CAD build for the part. Positions are in the model's coordinates, mm. Face numbers are marked on the shaded views. A direction names the side the tool comes from. Round coordinates to 2 decimals unless told otherwise and drop trailing zeros. Loops run counter-clockwise (first coordinate to the right, second up) from the corner with the lowest first, then second, coordinate; pieces in that order, holes last. Notation, with made-up numbers: M 23,64 L 34,64 A22 ccw 34,89 Z; hole C -24,-20 d10. An arc over 180 degrees is marked long. One line per item, written item: value. Start each with the question number.
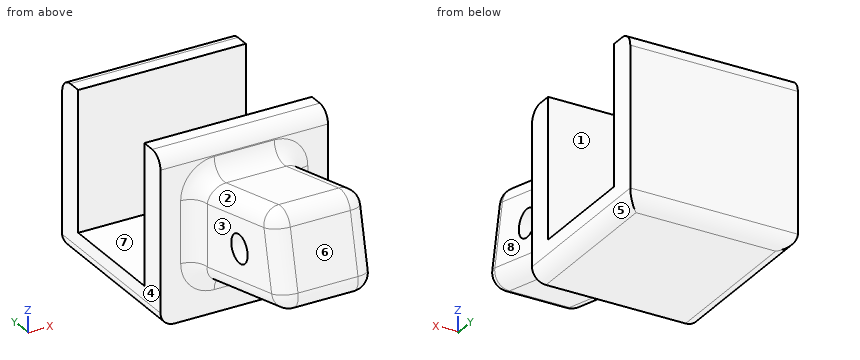
from build123d import *

# Parameters (mm, degrees)
F0_W      = 30
F0_H      = 30
F1_DEPTH  = 5
F2_W      = 30
F2_H      = 4.9
F3_DEPTH  = 25
F6_W      = 16.75
F6_H      = 16.75
F7_DEPTH  = 25
F7_FACE_W = 16.75
F7_FACE_H = 8.375
F9_R      = 3
F10_R     = 2.5
F12_R     = 2.5
F13_DEPTH = 16.75


# Not quite as in the source:
# - two fillets or chamfers of one size are made in one step
# - a feature names something its author has since deleted; it is built from what else it names


with BuildPart() as f1:
    # F0 (on Top) → F1 (new body)
    with BuildSketch(Plane.XY):
        with Locations((15, 15)):
            Rectangle(F0_W, F0_H)
    extrude(amount=F1_DEPTH)

    # F2 (on face) → F3 (join)
    with BuildSketch(Plane.XY.offset(5)):
        with Locations((15, 27.55)):
            Rectangle(F2_W, F2_H)
        with Locations((15, 2.45)):
            Rectangle(F2_W, F2_H)
    extrude(amount=F3_DEPTH)

    # F6 (on line) → F7 (join)
    with BuildSketch(Plane(origin=(0, -3.1696369631, 0.7026915972), x_dir=(1, 0, 0), z_dir=(0, -0.9762960071, 0.2164396139))):
        with Locations((15, 14.6444401068)):
            Rectangle(F6_W, F6_H)
    extrude(amount=F7_DEPTH)

    # F7_face (on face) → F8 (join, up to the next surface of F1)
    with BuildSketch(Plane(origin=(15, -0.9063408834, 10.9117604702), x_dir=(1, 0, 0), z_dir=(0, 0.9762960071, -0.2164396139))):
        Rectangle(F7_FACE_W, F7_FACE_H)
    extrude(until=Until.NEXT)

    # F9
    f9_edges = [f1.edges().sort_by_distance(p)[0] for p in [
        (6.625, -24.4074, 20.41099),
        (23.375, 0, 15),
        (23.375, -13.110041, 9.328085),
        (23.375, -24.4074, 20.41099),
        (23.375, -11.297359, 26.082905),
        (15, 0, 23.578341),
        (6.625, 0, 15),
        (15, 0, 6.421659),
        (6.625, -13.110041, 9.328085),
        (15, -26.220082, 12.234511),
        (15, -22.594718, 28.587469),
        (6.625, -11.297359, 26.082905),
    ]]
    fillet(f9_edges, radius=F9_R)

    # F10
    f10_edges = [f1.edges().sort_by_distance(p)[0] for p in [
        (15, 30, 30),
        (15, 0, 30),
        (15, 30, 0),
        (30, 15, 0),
        (0, 15, 0),
    ]]
    fillet(f10_edges, radius=F10_R)

    # F12 (on face) → F13 (cut, through all)
    with BuildSketch(Plane.YZ.offset(23.375)):
        with Locations((-12.8209375408, 17.8423334229)):
            Circle(F12_R)
    extrude(amount=-F13_DEPTH, mode=Mode.SUBTRACT)


solid = f1.part
(1) Slice it at B-B, the plane x = 14. List the corners of the cut face in (y, z).
(2) Flat gauge pins, fed straight in: P1, Ø2, axis at y = -12, z = 13.5, coming from the +X side (3 decimals); P2, Ø16.5, axis at y = -8.5, z = 18.5, coming from the +X side; P3, Ø1.5, axis at y = -7, z = 23, coming from the -X side. Where does each tip first touch, or does it go through?
(3) Mould opens along Y. For the marked faces 6, 7 and 8 say: pulls with the +Y half, pulls with the -Y half, needs draft (parallel to the pull), parting line crosses it, or undercut.
(4) Slice it at C-C, the plane z = 16. Count the separate pieces of the cut face and the enclosed holes in it, and give its area (3 significant figures).
(5) Probe L1, parallel to Y at x = 28, z = 27; L2, parallel to Y at x = 19.5, z = 20; L3, parallel to X at y = -6.5, z = 20.5 (3 decimals). List the from-to ranges inside material, lowest first.
(6) Which spindle directions (+Z, -Z, +X, -X, +Y, -Y) get a long thin tool onto all of the face, cutting with end or side? Do the marked faces 1, 2, 3, 4 and 5. Say none if no direction does.
(7) Slice it at A-A, the plane y = 21.5. List the corners of the cut face in (x, z).
Check result:
1. outline: M -25.57,15.16 A3 ccw -23.29,11.59 L -2.35,6.94 A3 cw 0,4.01 L 0,0 L 27.5,0 A2.5 ccw 30,2.5 L 30,27.5 A2.5 ccw 27.5,30 L 25.1,30 L 25.1,5 L 4.9,5 L 4.9,30 L 2.5,30 A2.5 ccw 0,27.5 L 0,27.32 A3 cw -3.65,24.39 L -19.67,27.94 A3 ccw -23.24,25.66 Z; hole C -12.82,17.84 d5
2. P1: stops at x = 23.375
2. P2: stops at x = 25.18
2. P3: stops at x = 6.63
3. face 6: pulls with the -Y half
3. face 7: undercut
3. face 8: needs draft
4. separate pieces: 3
4. enclosed holes: 0
4. area: 662 mm^2
5. L1: y = 0 to 4.9, 25.1 to 30
5. L2: y = -24.5 to -14.08, -11.56 to 4.9, 25.1 to 30
5. L3: x = 6.625 to 23.375
6. face 1: +Z, +X, -X
6. face 2: +Z, -X
6. face 3: +Z, -Z, -X, -Y
6. face 4: +Z, -Z, -X, +Y, -Y
6. face 5: -Z, +X, +Y, -Y
7. outline: M 0,2.5 A2.5 ccw 2.5,0 L 27.5,0 A2.5 ccw 30,2.5 L 30,5 L 0,5 Z
